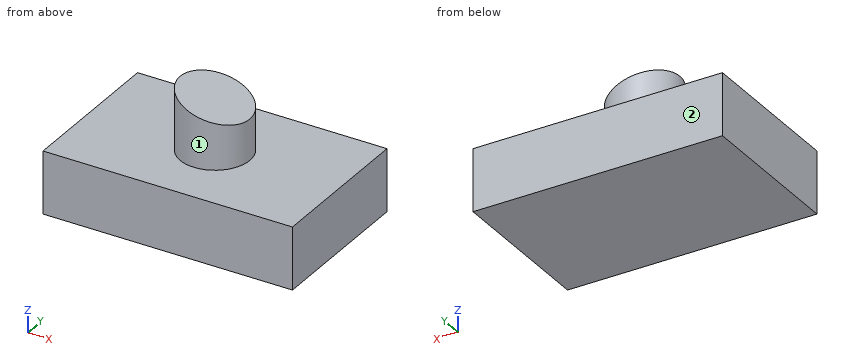
```python
from build123d import *

# Parameters (mm, degrees)
F0_W     = 101.6
F0_H     = 63.5
F2_DEPTH = 25.4
F1_R     = 14.185662
F3_DEPTH = 50.8
F5_DEPTH = 25.4


with BuildPart() as f2:
    # F0 (on Top) → F2 (new body)
    with BuildSketch(Plane.XY):
        Rectangle(F0_W, F0_H)
    extrude(amount=F2_DEPTH)

    # F1 (on face) → F3 (join)
    with BuildSketch(Plane.XY):
        Circle(F1_R)
    extrude(amount=F3_DEPTH)

    # F4 (on Front) → F5 (cut, symmetric)
    with BuildSketch(Plane.XZ):
        Polygon((14.185662, 50.8), (-14.185662, 50.8), (14.185662, 42.07477), align=None)
    extrude(amount=F5_DEPTH, both=True, mode=Mode.SUBTRACT)


solid = f2.part
```
Geometry: final body of the model. Coordinates: model frame, mm. Face numbers are marked on the shaded views. A direction names the side the tool comes from. Coordinates: 2 decimals unless noted, no trailing zeros. Order: outer loops, then holes, each group sorted by start corner. A loop starts at its lowest first (then second) coordinate and runs counter-clockwise, first axis right, second up. Notation, with made-up numbers: (7, 68) -> (42, 68) arc R26 ccw to (42, 99) -> close; hole circle Ø3 at (40.5, 60.25). An arc over 180 degrees is marked (long way). Write item = value, one per line.
(1) Cut plane B-B on x = -39. Return loops of the section in (y, z), plus the area to 3 significant figures.
Solved:
outline = (-31.75, 0) -> (31.75, 0) -> (31.75, 25.4) -> (-31.75, 25.4) -> close
area = 1,610 mm²
(2) Cut plane D-D on y = -24.5. Return loops of the section in (x, z), plus the area to 3 significant figures.
Solved:
outline = (-50.8, 0) -> (50.8, 0) -> (50.8, 25.4) -> (-50.8, 25.4) -> close
area = 2,580 mm²
(3) Cut plane C-C on z = 33. Return loops of the section in (x, y), plus the area to 3 significant figures.
Solved:
outline = circle Ø28.37 at (0, 0)
area = 632 mm²
(4) Line query: line 1 (Z direction, x = -34, y = 17); line 2 (X direction, y = 11, z = 40); line 3 (Y direction, x = 6, z = 37.5). Output: solid intervals per line, ascending.
Solved:
line_1 = 0 to 25.4
line_2 = -8.96 to 8.96
line_3 = -12.85 to 12.85
(5) Pin query (flat end, axial travel): pin 1 Ø10 at (x, y) = (22, -4.5) entering from +Z; pin 2 Ø2 at (x, z) = (-4.5, 33.5) entering from -Y. Return the tip coordinate at first contact, or that it passes through.
Solved:
pin_1 = 25.4
pin_2 = -13.75
(6) Cut plane A-A on y = 0. Return loops of the section in (x, z).
Solved:
outline = (-50.8, 0) -> (50.8, 0) -> (50.8, 25.4) -> (14.19, 25.4) -> (14.19, 42.07) -> (-14.19, 50.8) -> (-14.19, 25.4) -> (-50.8, 25.4) -> close
(7) Access query for the marked faces 1 and 2. Directions: +Z, -Z, +X, -X, +Y, -Y. A direction counts if a zero-diameter tool reaches every point of the face in a straight line with its end or side. Return the directions, or none.
Solved:
face_1 = +Z
face_2 = +Z, -Z, +X, -X, +Y
